Geometry check sheet. Reference: the model listing, model coordinates, mm. A direction names the side the tool comes from. Coordinates: 2 decimals unless noted, no trailing zeros. Order: outer loops, then holes, each group sorted by start corner. A loop starts at its lowest first (then second) coordinate and runs counter-clockwise, first axis right, second up. Notation, with made-up numbers: (8.5, 5) - (48.5, 5) arc R8 ccw to (48.5, 10) - close; hole circle Ø9 at (31, 31). An arc over 180 degrees is marked (long way). One line per item, written item: value. Start each with the question number.
```python
from build123d import *

# Parameters (mm, degrees)
BOSS_EXTRUDE1_DEPTH = 12
SKETCH2_R           = 3.1
BOSS_EXTRUDE2_DEPTH = 15
CUT_EXTRUDE1_START  = -50
CUT_EXTRUDE1_DEPTH  = 50
CUT_EXTRUDE2_START  = -15
CUT_EXTRUDE2_DEPTH  = 15
SKETCH5_W           = 7
SKETCH5_H           = 112.5
CUT_EXTRUDE3_DEPTH  = 12
SKETCH6_R           = 5.15
CUT_EXTRUDE4_DEPTH  = 2
FILLET1_R           = 4


with BuildPart() as part:
    # Sketch1 → Boss-Extrude1 (new body)
    with BuildSketch(Plane.XY):
        with BuildLine():
            Line((-5.64516129, 102.580645161), (-5.64516129, -27.419354839))
            ThreePointArc((-5.64516129, -27.419354839), (1.85483871, -34.919354839), (9.35483871, -27.419354839))
            Line((9.35483871, -27.419354839), (9.35483871, 102.580645161))
            ThreePointArc((9.35483871, 102.580645161), (1.85483871, 110.080645161), (-5.64516129, 102.580645161))
        make_face()
    extrude(amount=BOSS_EXTRUDE1_DEPTH)

    # Sketch2 → Boss-Extrude2 (add)
    with BuildSketch(Plane.XY.offset(12)):
        with Locations(Location((1.85483871, -27.419354839, 0), (0, 0, 180))):
            Circle(SKETCH2_R)
    extrude(amount=BOSS_EXTRUDE2_DEPTH)

    # Sketch3 → Cut-Extrude1 (cut)
    with BuildSketch(Plane.XY.offset(27).offset(CUT_EXTRUDE1_START)):
        with BuildLine():
            Line((0.166644408, -24.819354839), (3.543033011, -24.819354839))
            ThreePointArc((3.543033011, -24.819354839), (1.85483871, -30.519354839), (0.166644408, -24.819354839))
        make_face()
    extrude(amount=CUT_EXTRUDE1_DEPTH, mode=Mode.SUBTRACT)

    # Sketch4 → Cut-Extrude2 (cut)
    with BuildSketch(Plane.XY.offset(27).offset(CUT_EXTRUDE2_START)):
        with BuildLine():
            Line((0.166644408, -24.819354839), (3.543033011, -24.819354839))
            ThreePointArc((3.543033011, -24.819354839), (1.85483871, -24.319354839), (0.166644408, -24.819354839))
        make_face()
    extrude(amount=CUT_EXTRUDE2_DEPTH, mode=Mode.SUBTRACT)

    # Sketch5 → Cut-Extrude3 (cut)
    with BuildSketch(Plane.XY.offset(12)):
        with Locations((1.85483871, 36.330645161)):
            Rectangle(SKETCH5_W, SKETCH5_H)
    extrude(amount=-CUT_EXTRUDE3_DEPTH, mode=Mode.SUBTRACT)

    # Sketch6 → Cut-Extrude4 (cut)
    with BuildSketch(Plane.ZY.offset(5.64516129)):
        with Locations(Location((6, 78.768969581, 0), (0, 0, 270))):
            Circle(SKETCH6_R)
        with Locations(Location((6, 53.768969581, 0), (0, 0, 270))):
            Circle(SKETCH6_R)
        with Locations(Location((6, 28.768969581, 0), (0, 0, 270))):
            Circle(SKETCH6_R)
    extrude(amount=-CUT_EXTRUDE4_DEPTH, mode=Mode.SUBTRACT)

    # Fillet1
    # the kernel refuses this fillet: 4 mm, written as the material it adds along each edge
    with BuildSketch(Plane(origin=(-1.64516129, -19.919354839, 12), x_dir=(0, 1, 0), z_dir=(0, 0, -1)), Plane(origin=(5.35483871, -19.919354839, 12), x_dir=(-1, 0, 0), z_dir=(0, 0, -1)), Plane(origin=(5.35483871, 92.580645161, 12), x_dir=(0, -1, 0), z_dir=(0, 0, -1))) as fillet1_piece_1:
        with BuildLine():
            CenterArc((FILLET1_R, FILLET1_R), FILLET1_R, 180, 90)
            Line((0, FILLET1_R), (0, 0))
            Line((0, 0), (FILLET1_R, 0))
        make_face()
    extrude(amount=12)
    with BuildSketch(Plane(origin=(-1.64516129, 92.580645161, 12), x_dir=(0, -1, 0), z_dir=(0, 0, -1))) as fillet1_piece_2:
        with BuildLine():
            CenterArc((FILLET1_R, -FILLET1_R), FILLET1_R, 90, 90)
            Line((0, -FILLET1_R), (0, 0))
            Line((0, 0), (FILLET1_R, 0))
        make_face()
    extrude(amount=12)


solid = part.part
```
Q1. Cross-section at A-A, the plane y = 61. Enter the section's corners in (x, z), and give its area (3 significant figures).
Q2. Material ranges on probe 1 along X at (y, z) = (44, 10); probe 2 along X at (y, z) = (75, 8.75); probe 3 along Y at (x, z) = (4.5, 7), recorded low to high.
Q3. Gauge pin test, flat ends, axial feed: P1, Ø6, axis at y = 78.77, z = 6, coming from the -X side; P2, Ø5, axis at x = 1, y = 16, coming from the +Z side; P3, Ø3, axis at x = -2.5, z = 3, coming from the +Y side. Record the tip position at first contact, or that the pin passes through.
Q4. Set-up check for faces 4 (the cylindrical face through (-4.659, 83.914, 6.226)), 5 (the cylindrical face through (4.381, -18.535, 6.084)), 6 (the flat face through (-5.645, 38, 6)): record each of +Z, -Z, +X, -X, +Y, -Y from which the full face is reachable in a straight line by a thin tool's end or side.
Q5. Release check for a two-part mould opening along Y. For faces 1 (the cylindrical face through (4.328, 91.257, 6.084)), 2 (the cylindrical face through (2.02, 110.08, 5.92)), 3 (the flat face through (-3, 37, 0)) record: released by +Y, released by -Y, zero draft, split by the parting line, or undercut.
Q6. Cross-section at B-B, the plane z = 6. Enter the section's corners in (x, y), and give its area (3 significant figures).
Check result:
1. outline: (-5.65, 0) - (-1.65, 0) - (-1.65, 12) - (-5.65, 12) - close; (5.35, 0) - (9.35, 0) - (9.35, 12) - (5.35, 12) - close
1. area: 96.0 mm2
2. probe 1: x = -5.65 to -1.65, 5.35 to 9.35
2. probe 2: x = -3.65 to -1.65, 5.35 to 9.35
2. probe 3: y = -34.44 to -29.04, -25.8 to -18.39, 91.05 to 109.6
3. P1: stops at x = -3.65
3. P2: passes through
3. P3: stops at y = 109.52
4. face 4: -X
4. face 5: +Z, -Z
4. face 6: +Z, -Z, -X, +Y, -Y
5. face 1: undercut
5. face 2: released by +Y
5. face 3: zero draft
6. outline: (-5.65, -27.42) arc R7.5 ccw to (9.35, -27.42) - (9.35, 102.58) arc R7.5 ccw to (-5.65, 102.58) - (-5.65, 83.92) - (-3.65, 83.92) - (-3.65, 73.62) - (-5.65, 73.62) - (-5.65, 58.92) - (-3.65, 58.92) - (-3.65, 48.62) - (-5.65, 48.62) - (-5.65, 33.92) - (-3.65, 33.92) - (-3.65, 23.62) - (-5.65, 23.62) - close; hole (-1.65, -15.92) arc R4 ccw to (1.85, -19.89) arc R4 ccw to (5.35, -15.92) - (5.35, 88.58) arc R4 ccw to (1.85, 92.55) arc R4 ccw to (-1.65, 88.58) - close; hole (0.17, -24.82) arc R3.1 ccw (long way) to (3.54, -24.82) - close
6. area: 1,260 mm2
